Design review of the part built by this model. Coordinates are the model's own, in mm. Face numbers are marked on the shaded views. Coordinates: 2 decimals unless noted, no trailing zeros. Loops run counter-clockwise (first coordinate to the right, second up) from the corner with the lowest first, then second, coordinate; pieces in that order, holes last. Notation, with made-up numbers: (43, -29.75) - (83, -29.75) arc R9 ccw to (83, -25.75) - close; hole circle Ø8 at (36, 33.25). An arc over 180 degrees is marked (long way). Use one line per item in the form item = value. Start each with the question number.
(1) For L1, parallel to Y at x = -51, z = 6.9; L2, parallel to X at y = 2.5, z = 6; L3, parallel to Y at x = -2.5, z = 2.25, list the stretches that pass through material, from the lowest coordinate up.
(2) Clearance check with flat-ended pins moving along their axes: pin 1 Ø0.9 at (x, y) = (-41.5, 18) entering from +Z; pin 2 Ø6 at (x, y) = (-24.5, 11.5) entering from -Z. State where each tip first meets the part, or that it passes through.
(3) Add section A-A (z = 2). State the section outline as (x, y) points.
(4) Add section B-B (x = -9). State the section outline as (y, z) points, plus the area to 3 significant figures.
(5) Add section C-C (z = 6.5). Count the separate pieces of the cut face and the enclosed holes in it, plus the area to 3 significant figures.
(6) The part is to be moulded in two halves that separate along Y. For the marked faces 1, 2 and 3, say which applies: pulls with the +Y half, pulls with the -Y half, needs draft (parallel to the pull), parting line crosses it, or undercut.
(7) Add section D-D (y = 2.5). State the section outline as (x, z) points.
```python
from build123d import *

# Parameters (mm, degrees)
ESQUISSE1_W             = 60
ESQUISSE1_H             = 20
BOSS_EXTRU_1_DEPTH      = 7.8
ESQUISSE2_W             = 60
ESQUISSE2_H             = 10
ENL_V_MAT_EXTRU_1_DEPTH = 3.3
ESQUISSE4_R             = 1.5
ENL_V_MAT_EXTRU_2_DEPTH = 3


with BuildPart() as part:
    # Esquisse1 → Boss.-Extru.1 (new body)
    with BuildSketch(Plane.XY):
        with Locations((-30, 10)):
            Rectangle(ESQUISSE1_W, ESQUISSE1_H)
    extrude(amount=BOSS_EXTRU_1_DEPTH)

    # Esquisse2 → Enlèv. mat.-Extru.1 (cut)
    with BuildSketch(Plane(origin=(0, 0, 0), x_dir=(-1, 0, 0), z_dir=(0, 0, -1))):
        with Locations((30, 10)):
            Rectangle(ESQUISSE2_W, ESQUISSE2_H)
    extrude(amount=-ENL_V_MAT_EXTRU_1_DEPTH, mode=Mode.SUBTRACT)

    # Esquisse4 → Enlèv. mat.-Extru.2 (cut)
    with BuildSketch(Plane.XY.offset(7.8)):
        with Locations((-51, 17.5)):
            Circle(ESQUISSE4_R)
        with Locations((-41, 17.5)):
            Circle(ESQUISSE4_R)
        with Locations((-19, 17.5)):
            Circle(ESQUISSE4_R)
        with Locations((-9, 17.5)):
            Circle(ESQUISSE4_R)
        with Locations(Location((-9, 2.5, 0), (0, 0, 180))):
            Circle(ESQUISSE4_R)
        with Locations(Location((-19, 2.5, 0), (0, 0, 180))):
            Circle(ESQUISSE4_R)
        with Locations(Location((-41, 2.5, 0), (0, 0, 180))):
            Circle(ESQUISSE4_R)
        with Locations(Location((-51, 2.5, 0), (0, 0, 180))):
            Circle(ESQUISSE4_R)
    extrude(amount=-ENL_V_MAT_EXTRU_2_DEPTH, mode=Mode.SUBTRACT)


solid = part.part
```
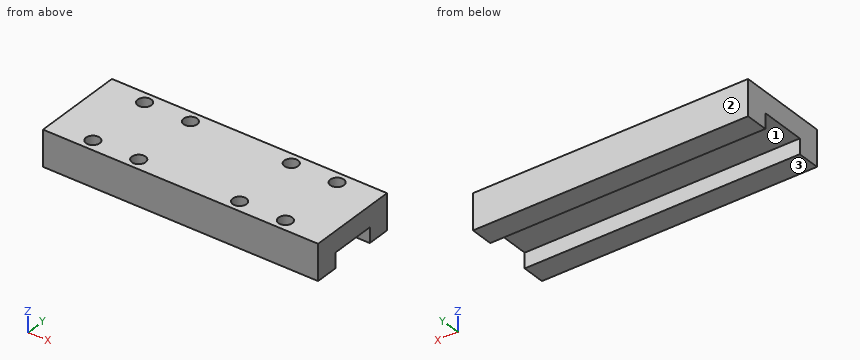
Computed values:
q1.L1 = 0 to 1, 4 to 16, 19 to 20
q1.L2 = -60 to -52.5, -49.5 to -42.5, -39.5 to -20.5, -17.5 to -10.5, -7.5 to 0
q1.L3 = 0 to 5, 15 to 20
q2.pin_1 = 4.8
q2.pin_2 = 3.3
q3.outline = (-60, 0) - (0, 0) - (0, 5) - (-60, 5) - close; (-60, 15) - (0, 15) - (0, 20) - (-60, 20) - close
q4.outline = (0, 0) - (5, 0) - (5, 3.3) - (15, 3.3) - (15, 0) - (20, 0) - (20, 7.8) - (19, 7.8) - (19, 4.8) - (16, 4.8) - (16, 7.8) - (4, 7.8) - (4, 4.8) - (1, 4.8) - (1, 7.8) - (0, 7.8) - close
q4.area = 105 mm^2
q5.separate_pieces = 1
q5.enclosed_holes = 8
q5.area = 1,140 mm^2
q6.face_1 = undercut
q6.face_2 = pulls with the +Y half
q6.face_3 = needs draft
q7.outline = (-60, 0) - (0, 0) - (0, 7.8) - (-7.5, 7.8) - (-7.5, 4.8) - (-10.5, 4.8) - (-10.5, 7.8) - (-17.5, 7.8) - (-17.5, 4.8) - (-20.5, 4.8) - (-20.5, 7.8) - (-39.5, 7.8) - (-39.5, 4.8) - (-42.5, 4.8) - (-42.5, 7.8) - (-49.5, 7.8) - (-49.5, 4.8) - (-52.5, 4.8) - (-52.5, 7.8) - (-60, 7.8) - close
